from build123d import *

# Parameters (mm, degrees)
SKETCH1_W               = 342.9
SKETCH1_H               = 101.6
BOSS_EXTRUDE1_DEPTH     = 9.525
CUT_EXTRUDE1_DEPTH      = 208.28
CUT_EXTRUDE1_DEPTH_BACK = 9.525
CUT_EXTRUDE1_START      = 60.325
SKETCH2_W               = 1.5875
SKETCH2_H               = 50.8
CUT_EXTRUDE4_DEPTH      = 358.76206566
CUT_EXTRUDE4_DEPTH_BACK = 358.76206566
SKETCH3_R               = 6.35
SKETCH5_W               = 50.8
SKETCH5_H               = 101.6
CUT_EXTRUDE5_DEPTH      = 1.5875
M5_CLEARANCE_HOLE1_D    = 5.5


with BuildPart() as part:
    # Sketch1 → Boss-Extrude1 (new body)
    with BuildSketch(Plane.XY):
        with Locations((171.45, 50.8)):
            Rectangle(SKETCH1_W, SKETCH1_H)
    extrude(amount=BOSS_EXTRUDE1_DEPTH)

    # Sketch2 → Cut-Extrude1 (cut, two sides: drawn at the far end of the back side and taken through both)
    with BuildSketch(Plane(origin=(0, 0, 0), x_dir=(0, 0, -1), z_dir=(1, 0, 0)).offset(CUT_EXTRUDE1_START - CUT_EXTRUDE1_DEPTH_BACK)):
        with Locations((-0.79375, 50.8)):
            Rectangle(SKETCH2_W, SKETCH2_H)
    extrude(amount=CUT_EXTRUDE1_DEPTH + CUT_EXTRUDE1_DEPTH_BACK, mode=Mode.SUBTRACT)

    # Sketch3 → Cut-Extrude4 (cut, two sides: drawn at the far end of the back side and taken through both)
    with BuildSketch(Plane(origin=(0, 0, 0), x_dir=(-1, 0, 0), z_dir=(0, 0, -1)).offset(-CUT_EXTRUDE4_DEPTH_BACK)):
        with Locations((-12.7, 88.9)):
            Circle(SKETCH3_R)
        with Locations((-114.3, 88.9)):
            Circle(SKETCH3_R)
        with Locations((-114.3, 12.7)):
            Circle(SKETCH3_R)
        with Locations((-12.7, 12.7)):
            Circle(SKETCH3_R)
    extrude(amount=CUT_EXTRUDE4_DEPTH + CUT_EXTRUDE4_DEPTH_BACK, mode=Mode.SUBTRACT)

    # Sketch5 → Cut-Extrude5 (cut)
    with BuildSketch(Plane(origin=(0, 0, 0), x_dir=(-1, 0, 0), z_dir=(0, 0, -1))):
        with Locations((-76.2, 50.8)):
            Rectangle(SKETCH5_W, SKETCH5_H)
    extrude(amount=-CUT_EXTRUDE5_DEPTH, mode=Mode.SUBTRACT)

    # M5 Clearance Hole1 (through all)
    with Locations(Plane.XY.offset(9.525)):
        with Locations((328.2696, 62.9412), (328.2696, 39.9288), (288.2646, 39.9288), (288.2646, 62.9412)):
            Hole(M5_CLEARANCE_HOLE1_D / 2)


solid = part.part
Verification items for the finished model (mm, model axes). Coordinates: 2 decimals unless noted, no trailing zeros. Order: outer loops, then holes, each group sorted by start corner. A loop starts at its lowest first (then second) coordinate and runs counter-clockwise, first axis right, second up.
Item 1: Section check B-B, the plane y = 12.7. Give the number of separate pieces and of enclosed holes in the cut face, then the cut area to 3 significant figures.
Filled in:
separate pieces: 3
enclosed holes: 0
area: 2,940 mm2
Item 2: Depth check by flat-ended pin: pin 1 (10 mm diameter, centred on x = 12.7, y = 88.9, fed in from -Z). Enter the tip coordinate at first touch or a pass-through.
Filled in:
pin 1: passes through
Item 3: Release check for a two-part mould opening along X. For faces 1 (the face through (110.886, 94.254, 4.829)), 2 (the face through (169, 101.6, 5)), 3 (the face through (0, 50, 5)) record: +X half, -X half, draft (parallel to the pull), parting line (faces both ways), or undercut.
Filled in:
face 1: undercut
face 2: draft
face 3: -X half
Item 4: Material ranges on L1, parallel to Y at x = 12.7, z = 2; L2, parallel to X at y = 63.5, z = 4; L3, parallel to X at y = 88.9, z = 4.25, recorded low to high.
Filled in:
L1: y = 0 to 6.35, 19.05 to 82.55, 95.25 to 101.6
L2: x = 0 to 285.57, 290.96 to 325.58, 330.96 to 342.9
L3: x = 0 to 6.35, 19.05 to 107.95, 120.65 to 342.9
Item 5: Section check A-A, the plane x = 12.7. Enter the section's corners in (y, z) (3 decimals).
Filled in:
outline: (0, 0) - (6.35, 0) - (6.35, 9.525) - (0, 9.525) - close; (19.05, 0) - (82.55, 0) - (82.55, 9.525) - (19.05, 9.525) - close; (95.25, 0) - (101.6, 0) - (101.6, 9.525) - (95.25, 9.525) - close
